Part model, mm, in its own coordinate system. A direction names the side the tool comes from. Coordinates: 2 decimals unless noted, no trailing zeros. Order: outer loops, then holes, each group sorted by start corner. A loop starts at its lowest first (then second) coordinate and runs counter-clockwise, first axis right, second up. Notation, with made-up numbers: (8.25, 16) - (38.25, 16) arc R20 cw to (38.25, 39) - close; hole circle Ø2 at (28, 34.5). An arc over 180 degrees is marked (long way). Use a Markdown table: item, result. Add a question column.
1) Wall check: L1, parallel to X at y = 77.5, z = -5.5; L2, parallel to Y at x = 9, z = -4.75; L3, parallel to X at y = 9, z = -3.25. Give the ranges that are in metal, low to high. Write a range as [from, to].
2) Two-plate mould, pull along X, no slides. Class faces 4 (the face through (1, 80, -1)), 5 (the face through (0, 79, -5)), 6 (the face through (9, 125, -4)), 7 (the face through (13, 87, -1)): +X half, -X half, draft (parallel to the pull), parting line (faces both ways), or undercut.
3) Drop a flat-ended pin along its axis: P1, Ø6.5, axis at x = 62, y = 128, coming from the +Z side. Give the stop position or say it passes through.
4) Saw through at A-A on y = 87.5. List the corners of the cut face in (x, z).
5) Saw through at C-C on y = 21.5. List the corners of the cut face in (x, z).
6) Tool access for faces 1 (the face through (35, 0, -5)), 2 (the face through (34.527, 125.495, -5.563)), 3 (the face through (53, 126, -0.5)): list every direction of +Z, -Z, +X, -X, +Y, -Y with a clear straight run to the whole face (end or side of a thin tool).
7) Saw through at B-B on x = 34.5. List the corners of the cut face in (y, z).
```python
from build123d import *

# Parameters (mm, degrees)
CROQUIS1_W              = 70
CROQUIS1_H              = 160
SALIENTE_EXTRUIR1_DEPTH = 10
VACIADO1_T              = -3
CROQUIS2_W              = 70
CROQUIS2_H              = 160
CROQUIS2_W_2            = 66
CROQUIS2_H_2            = 156
CORTAR_EXTRUIR1_DEPTH   = 1
SALIENTE_EXTRUIR2_DEPTH = 6
CORTAR_EXTRUIR2_START   = -6
CORTAR_EXTRUIR2_DEPTH   = 6
CROQUIS5_R              = 3
CROQUIS5_R_2            = 1.25
SALIENTE_EXTRUIR3_DEPTH = 6.5
CROQUIS6_R              = 3
CROQUIS6_R_2            = 1.25
SALIENTE_EXTRUIR4_DEPTH = 6.5


with BuildPart() as part:
    # Croquis1 → Saliente-Extruir1 (new body)
    with BuildSketch(Plane.XY):
        with Locations((35, 80)):
            Rectangle(CROQUIS1_W, CROQUIS1_H)
    extrude(amount=-SALIENTE_EXTRUIR1_DEPTH)

    # Vaciado1
    vaciado1_openings = [part.faces().sort_by_distance(p)[0] for p in [
        (35, 80, 0),
    ]]
    offset(amount=VACIADO1_T, openings=vaciado1_openings, kind=Kind.INTERSECTION)

    # Croquis2 → Cortar-Extruir1 (cut)
    with BuildSketch(Plane.XY):
        with Locations((35, 80)):
            Rectangle(CROQUIS2_W, CROQUIS2_H)
        with Locations((35, 80)):
            Rectangle(CROQUIS2_W_2, CROQUIS2_H_2, mode=Mode.SUBTRACT)
    extrude(amount=-CORTAR_EXTRUIR1_DEPTH, mode=Mode.SUBTRACT)

    # Croquis3 → Saliente-Extruir2 (add)
    with BuildSketch(Plane.XY.offset(-7)):
        with BuildLine():
            Line((58, 104), (58, 64))
            ThreePointArc((58, 64), (35, 41), (12, 64))
            Line((12, 64), (12, 104))
            ThreePointArc((12, 104), (35, 127), (58, 104))
        make_face()
        with BuildLine():
            Line((56.5, 104), (56.5, 64))
            ThreePointArc((56.5, 64), (35, 42.5), (13.5, 64))
            Line((13.5, 64), (13.5, 104))
            ThreePointArc((13.5, 104), (35, 125.5), (56.5, 104))
        make_face(mode=Mode.SUBTRACT)
    extrude(amount=SALIENTE_EXTRUIR2_DEPTH)

    # Croquis4 → Cortar-Extruir2 (cut)
    with BuildSketch(Plane.XY.offset(-7).offset(CORTAR_EXTRUIR2_START)):
        with BuildLine():
            Line((56.5, 104), (56.5, 64))
            ThreePointArc((56.5, 64), (35, 42.5), (13.5, 64))
            Line((13.5, 64), (13.5, 104))
            ThreePointArc((13.5, 104), (35, 125.5), (56.5, 104))
        make_face()
    extrude(amount=CORTAR_EXTRUIR2_DEPTH, mode=Mode.SUBTRACT)

    # Croquis5 → Saliente-Extruir3 (add)
    # profile 1 of 4: a face of its own
    with BuildSketch(Plane.XY.offset(-7)):
        with Locations(Location((17, 124.5, 0), (0, 0, 180))):
            Circle(CROQUIS5_R)
        with Locations(Location((17, 124.5, 0), (0, 0, 180))):
            Circle(CROQUIS5_R_2, mode=Mode.SUBTRACT)
    # profile 2 of 4: a face of its own
    with BuildSketch(Plane.XY.offset(-7)):
        with Locations(Location((53, 124.5, 0), (0, 0, 180))):
            Circle(CROQUIS5_R)
        with Locations(Location((53, 124.5, 0), (0, 0, 180))):
            Circle(CROQUIS5_R_2, mode=Mode.SUBTRACT)
    # profile 3 of 4: a face of its own
    with BuildSketch(Plane.XY.offset(-7)):
        with Locations(Location((17, 43.5, 0), (0, 0, 180))):
            Circle(CROQUIS5_R)
        with Locations(Location((17, 43.5, 0), (0, 0, 180))):
            Circle(CROQUIS5_R_2, mode=Mode.SUBTRACT)
    # profile 4 of 4: a face of its own
    with BuildSketch(Plane.XY.offset(-7)):
        with Locations(Location((53, 43.5, 0), (0, 0, 180))):
            Circle(CROQUIS5_R)
        with Locations(Location((53, 43.5, 0), (0, 0, 180))):
            Circle(CROQUIS5_R_2, mode=Mode.SUBTRACT)
    extrude(amount=SALIENTE_EXTRUIR3_DEPTH)

    # Croquis6 → Saliente-Extruir4 (add)
    # profile 1 of 4: a face of its own
    with BuildSketch(Plane.XY.offset(-7)):
        with Locations(Location((9, 9, 0), (0, 0, 180))):
            Circle(CROQUIS6_R)
        with Locations(Location((9, 9, 0), (0, 0, 180))):
            Circle(CROQUIS6_R_2, mode=Mode.SUBTRACT)
    # profile 2 of 4: a face of its own
    with BuildSketch(Plane.XY.offset(-7)):
        with Locations(Location((61, 9, 0), (0, 0, 180))):
            Circle(CROQUIS6_R)
        with Locations(Location((61, 9, 0), (0, 0, 180))):
            Circle(CROQUIS6_R_2, mode=Mode.SUBTRACT)
    # profile 3 of 4: a face of its own
    with BuildSketch(Plane.XY.offset(-7)):
        with Locations(Location((9, 128, 0), (0, 0, 180))):
            Circle(CROQUIS6_R)
        with Locations(Location((9, 128, 0), (0, 0, 180))):
            Circle(CROQUIS6_R_2, mode=Mode.SUBTRACT)
    # profile 4 of 4: a face of its own
    with BuildSketch(Plane.XY.offset(-7)):
        with Locations(Location((61, 128, 0), (0, 0, 180))):
            Circle(CROQUIS6_R)
        with Locations(Location((61, 128, 0), (0, 0, 180))):
            Circle(CROQUIS6_R_2, mode=Mode.SUBTRACT)
    extrude(amount=SALIENTE_EXTRUIR4_DEPTH)


solid = part.part
```
Results are:
| question | item | result |
|---|---|---|
| 1 | L1 | [0, 3], [12, 13.5], [56.5, 58], [67, 70] |
| 1 | L2 | [0, 3], [6, 7.75], [10.25, 12], [125, 126.75], [129.25, 131], [157, 160] |
| 1 | L3 | [0, 3], [6, 7.75], [10.25, 12], [58, 59.75], [62.25, 64], [67, 70] |
| 2 | face 4 | draft |
| 2 | face 5 | -X half |
| 2 | face 6 | undercut |
| 2 | face 7 | undercut |
| 3 | P1 | z = -0.5 |
| 4 | outline | (0, -10) - (13.5, -10) - (13.5, -1) - (12, -1) - (12, -7) - (3, -7) - (3, 0) - (2, 0) - (2, -1) - (0, -1) - close; (56.5, -10) - (70, -10) - (70, -1) - (68, -1) - (68, 0) - (67, 0) - (67, -7) - (58, -7) - (58, -1) - (56.5, -1) - close |
| 5 | outline | (0, -10) - (70, -10) - (70, -1) - (68, -1) - (68, 0) - (67, 0) - (67, -7) - (3, -7) - (3, 0) - (2, 0) - (2, -1) - (0, -1) - close |
| 6 | face 1 | +Z, -Z, +X, -X, -Y |
| 6 | face 2 | +Z, -Z |
| 6 | face 3 | +Z |
| 7 | outline | (0, -10) - (42.51, -10) - (42.51, -1) - (41.01, -1) - (41.01, -7) - (3, -7) - (3, 0) - (2, 0) - (2, -1) - (0, -1) - close; (125.49, -10) - (160, -10) - (160, -1) - (158, -1) - (158, 0) - (157, 0) - (157, -7) - (126.99, -7) - (126.99, -1) - (125.49, -1) - close |
